Source: CAD feature listing. Evaluate the final solid. Frame: model axes, mm. Face numbers are marked on the shaded views. Give positions to 0.01 mm unless a question says otherwise; leave off trailing zeros. Write each loop counter-clockwise with the first axis right and the second up, starting at its lowest first coordinate (ties: lowest second). Pieces come first, ordered by that corner, then holes. Notation, with made-up numbers: (28.5, 33) -> (54.5, 33) arc R29 ccw to (54.5, 59) -> close; hole circle Ø9 at (-6.5, 56). An arc over 180 degrees is marked (long way). Use a Markdown table: item, result. Add a question column.
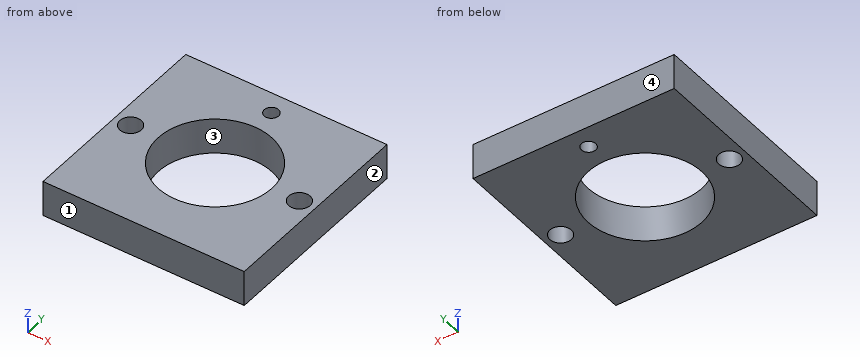
```python
from build123d import *

# Parameters (mm, degrees)
F0_W     = 62
F0_H     = 62
F1_DEPTH = 11
F3_D     = 6.6
F5_D     = 4.4
F6_R     = 17.5
F7_DEPTH = 11.001


with BuildPart() as f1:
    # F0 (on Top) → F1 (new body)
    with BuildSketch(Plane.XY):
        with Locations((31, 31)):
            Rectangle(F0_W, F0_H)
    extrude(amount=F1_DEPTH)

    # F3 (through all)
    with Locations(Plane.XY.offset(11)):
        with Locations((5, 31), (57, 31)):
            Hole(F3_D / 2)

    # F5 (through all)
    with Locations(Plane.XY.offset(11)):
        with Locations((31, 55.5)):
            Hole(F5_D / 2)

    # F6 (on face) → F7 (cut, through all)
    with BuildSketch(Plane.XY.offset(11)):
        with Locations((31, 31)):
            Circle(F6_R)
    extrude(amount=-F7_DEPTH, mode=Mode.SUBTRACT)


solid = f1.part
```
(1) Material intervals for L1, parallel to Y at x = 31, z = 4; L2, parallel to Y at x = 57, z = 4.5; L3, parallel to X at y = 27.5, z = 2.75, sorted ascending.
(2) Cut plane D-D on z = 9. Return the cut outline in (x, y).
(3) Cut plane B-B on y = 55.5. Return the cut outline in (x, z), then the cut area to 3 significant figures.
(4) Cut plane A-A on x = 5. Return the cut outline in (y, z).
(5) Mould query, pull axis Y, two halves, no side actions, for the marked faces 1, 2, 3 and 4. Classes: +Y half, -Y half, draft (parallel to the pull), parting line (faces both ways), or undercut.
(6) First-contact query: pin 1 Ø7 at (x, y) = (31, 55.5) entering from +Z. Flat tip, straight axial feed; report the tip coordinate or a pass-through.
(7) Cut plane C-C on x = 31. Return the cut outline in (y, z), then the cut area to 3 significant figures.
Output:
| question | item | result |
|---|---|---|
| 1 | L1 | 0 to 13.5, 48.5 to 53.3, 57.7 to 62 |
| 1 | L2 | 0 to 27.7, 34.3 to 62 |
| 1 | L3 | 0 to 13.85, 48.15 to 62 |
| 2 | outline | (0, 0) -> (62, 0) -> (62, 62) -> (0, 62) -> close; hole circle Ø6.6 at (5, 31); hole circle Ø35 at (31, 31); hole circle Ø4.4 at (31, 55.5); hole circle Ø6.6 at (57, 31) |
| 3 | outline | (0, 0) -> (28.8, 0) -> (28.8, 11) -> (0, 11) -> close; (33.2, 0) -> (62, 0) -> (62, 11) -> (33.2, 11) -> close |
| 3 | area | 634 mm^2 |
| 4 | outline | (0, 0) -> (27.7, 0) -> (27.7, 11) -> (0, 11) -> close; (34.3, 0) -> (62, 0) -> (62, 11) -> (34.3, 11) -> close |
| 5 | face 1 | -Y half |
| 5 | face 2 | draft |
| 5 | face 3 | undercut |
| 5 | face 4 | +Y half |
| 6 | pin 1 | z = 11 |
| 7 | outline | (0, 0) -> (13.5, 0) -> (13.5, 11) -> (0, 11) -> close; (48.5, 0) -> (53.3, 0) -> (53.3, 11) -> (48.5, 11) -> close; (57.7, 0) -> (62, 0) -> (62, 11) -> (57.7, 11) -> close |
| 7 | area | 249 mm^2 |
